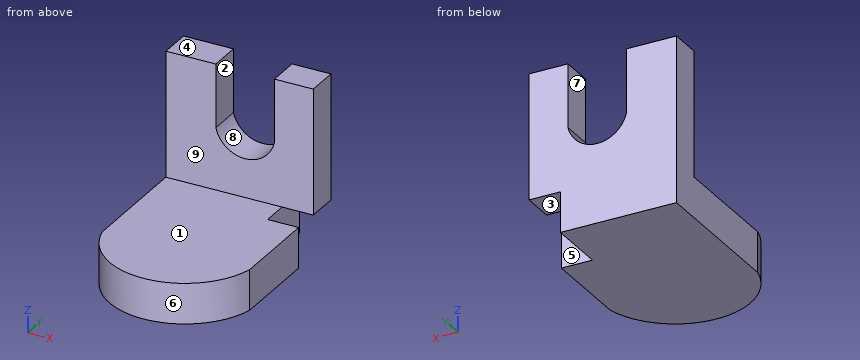
from build123d import *

# Parameters (mm, degrees)
F1_DEPTH = 12.7
F3_DEPTH = 10.16


with BuildPart() as f1:
    # F0 (on Top) → F1 (new body)
    with BuildSketch(Plane.XY):
        with BuildLine():
            Line((0, 27.773257), (-36.551334, 27.773257))
            Line((-36.551334, 27.773257), (-36.551334, -8.778076))
            ThreePointArc((-36.551334, -8.778076), (-13.38297, -27.332701), (9.785393, -8.778076))
            Line((9.785393, -8.778076), (9.785393, 19.426888))
            Line((9.785393, 19.426888), (0, 19.426888))
            Line((0, 19.426888), (0, 27.773257))
        make_face()
    extrude(amount=F1_DEPTH)

    # F2 (on face) → F3 (join)
    with BuildSketch(Plane(origin=(0, 27.773257, 0), x_dir=(-1, 0, 0), z_dir=(0, 1, 0))):
        with BuildLine():
            Line((0, 0), (36.551334, 0))
            Line((36.551334, 0), (36.551334, 52.096579))
            Line((36.551334, 52.096579), (20.838689, 52.096579))
            Line((20.838689, 52.096579), (20.838689, 32.179791))
            ThreePointArc((20.838689, 32.179791), (11.628905, 24.830871), (2.419121, 32.179791))
            Line((2.419121, 32.179791), (2.419121, 52.096579))
            Line((2.419121, 52.096579), (-9.817014, 52.096579))
            Line((-9.817014, 52.096579), (-9.817014, 12.7))
            Line((-9.817014, 12.7), (0, 12.7))
            Line((0, 12.7), (0, 0))
        make_face()
    extrude(amount=F3_DEPTH)


solid = f1.part
Check sheet for the modelled part. Datum: model origin and axes. Units: mm. Face numbers are marked on the shaded views. A direction names the side the tool comes from. Give positions to 0.01 mm unless a question says otherwise; leave off trailing zeros. Write each loop counter-clockwise with the first axis right and the second up, starting at its lowest first coordinate (ties: lowest second). Pieces come first, ordered by that corner, then holes. Notation, with made-up numbers: (-36.5, -4.5) -> (10.5, -4.5) arc R22 ccw to (10.5, 34.5) -> close; hole circle Ø7 at (-6.75, -12.75). An arc over 180 degrees is marked (long way). Write item = value, one per line.
Item 1: Scan lines: probe 1 along Z at (x, y) = (-26, 23.5); probe 2 along Y at (x, z) = (-25.5, 30.5); probe 3 along X at (y, z) = (32, 3). Record each from-to range of solid material in increasing order. Write a range as from..to.
Output:
probe_1 = 0..12.7
probe_2 = 27.77..37.93
probe_3 = -36.55..0
Item 2: Tool access check on the marked faces 1, 2, 3, 4 and 5. Record the directions out of +Z, -Z, +X, -X, +Y, -Y that give a thin tool (end or side, any length) a straight path to the whole face; none if there is none.
Output:
face_1 = +Z, +X, -X, -Y
face_2 = +Z, +Y, -Y
face_3 = -Z, +X, +Y
face_4 = +Z, +X, -X, +Y, -Y
face_5 = +Z, -Z, +X, +Y
Item 3: Sectioned sample at C-C on x = 3.5. Record the boundary of the cut face in (y, z).
Output:
outline = (-20.28, 0) -> (19.43, 0) -> (19.43, 12.7) -> (-20.28, 12.7) -> close; (27.77, 12.7) -> (37.93, 12.7) -> (37.93, 52.1) -> (27.77, 52.1) -> close
Item 4: Sectioned sample at B-B on y = 29. Record the boundary of the cut face in (x, z).
Output:
outline = (-36.55, 0) -> (0, 0) -> (0, 12.7) -> (9.82, 12.7) -> (9.82, 52.1) -> (-2.42, 52.1) -> (-2.42, 32.18) arc R9.45 cw to (-20.84, 32.18) -> (-20.84, 52.1) -> (-36.55, 52.1) -> close
Item 5: Sectioned sample at A-A on z = 42. Record the boundary of the cut face in (x, y), and give its area (3 significant figures).
Output:
outline = (-36.55, 27.77) -> (-20.84, 27.77) -> (-20.84, 37.93) -> (-36.55, 37.93) -> close; (-2.42, 27.77) -> (9.82, 27.77) -> (9.82, 37.93) -> (-2.42, 37.93) -> close
area = 284 mm^2
Item 6: Release check for a two-part mould opening along X. For the marked faces 6, 7, 8 and 9 record: +X half, -X half, draft (parallel to the pull), parting line (faces both ways), or undercut.
Output:
face_6 = parting line
face_7 = undercut
face_8 = undercut
face_9 = draft
Item 7: Sectioned sample at D-D on z = 9. Record the boundary of the cut face in (x, y).
Output:
outline = (-36.55, -8.78) arc R23.74 ccw to (9.79, -8.78) -> (9.79, 19.43) -> (0, 19.43) -> (0, 37.93) -> (-36.55, 37.93) -> close
Item 8: Gauge pin test, flat ends, axial feed: pin 1 (6.5 mm diameter, centred on y = 31, z = 7, fed in from +X); pin 2 (2 mm diameter, centred on x = -2.5, z = 17.5, fed in from -Y); pin 3 (5 mm diameter, centred on x = 5, z = 4, fed in from +Y). Record the tip position at first contact, or that the pin passes through.
Output:
pin_1 = 0
pin_2 = 27.77
pin_3 = 19.43
